from build123d import *

# Parameters (mm, degrees)
F0_R      = 40
F0_R_2    = 1.7
F1_DEPTH  = 14
F2_R      = 4.5
F2_R_2    = 1.7
F3_DEPTH  = 7
F4_R      = 4.5
F4_R_2    = 1.7
F5_DEPTH  = 4.6
F6_R      = 12.5
F7_DEPTH  = 8
F8_R      = 1
F10_R     = 32.1563127089
F11_DEPTH = 0.3


with BuildPart() as f1:
    # F0 (on Top) → F1 (new body)
    with BuildSketch(Plane.XY):
        Circle(F0_R)
        with Locations((-15.4640459878, -31.3984598617)):
            Circle(F0_R_2, mode=Mode.SUBTRACT)
        with Locations((-11.9054035877, -24.7893397535)):
            Circle(F0_R_2, mode=Mode.SUBTRACT)
        with Locations((-34.9238868738, -2.3069732602)):
            Circle(F0_R_2, mode=Mode.SUBTRACT)
        with Locations((-27.4208997634, -2.0842879275)):
            Circle(F0_R_2, mode=Mode.SUBTRACT)
        with Locations((19.4598408861, -29.0914866016)):
            Circle(F0_R_2, mode=Mode.SUBTRACT)
        with Locations((15.5154961757, -22.705051826)):
            Circle(F0_R_2, mode=Mode.SUBTRACT)
        with Locations((-15.5154961757, 22.705051826)):
            Circle(F0_R_2, mode=Mode.SUBTRACT)
        with Locations((-19.4598408861, 29.0914866016)):
            Circle(F0_R_2, mode=Mode.SUBTRACT)
        with Locations((27.4208997634, 2.0842879275)):
            Circle(F0_R_2, mode=Mode.SUBTRACT)
        with Locations((34.9238868738, 2.3069732602)):
            Circle(F0_R_2, mode=Mode.SUBTRACT)
        with Locations((11.9054035877, 24.7893397535)):
            Circle(F0_R_2, mode=Mode.SUBTRACT)
        with Locations((15.4640459878, 31.3984598617)):
            Circle(F0_R_2, mode=Mode.SUBTRACT)
    extrude(amount=F1_DEPTH)

    # F2 (on face) → F3 (cut)
    with BuildSketch(Plane.XY.offset(14)):
        with Locations((-15.5154961757, 22.705051826)):
            Circle(F2_R)
        with Locations((-15.5154961757, 22.705051826)):
            Circle(F2_R_2, mode=Mode.SUBTRACT)
        with Locations((-27.4208997634, -2.0842879275)):
            Circle(F2_R)
        with Locations((-27.4208997634, -2.0842879275)):
            Circle(F2_R_2, mode=Mode.SUBTRACT)
        with Locations((-11.9054035877, -24.7893397535)):
            Circle(F2_R)
        with Locations((-11.9054035877, -24.7893397535)):
            Circle(F2_R_2, mode=Mode.SUBTRACT)
        with Locations((15.5154961757, -22.705051826)):
            Circle(F2_R)
        with Locations((15.5154961757, -22.705051826)):
            Circle(F2_R_2, mode=Mode.SUBTRACT)
        with Locations((27.4208997634, 2.0842879275)):
            Circle(F2_R)
        with Locations((27.4208997634, 2.0842879275)):
            Circle(F2_R_2, mode=Mode.SUBTRACT)
        with Locations((11.9054035877, 24.7893397535)):
            Circle(F2_R)
        with Locations((11.9054035877, 24.7893397535)):
            Circle(F2_R_2, mode=Mode.SUBTRACT)
    extrude(amount=-F3_DEPTH, mode=Mode.SUBTRACT)

    # F4 (on face) → F5 (cut)
    with BuildSketch(Plane(origin=(0, 0, 0), x_dir=(1, 0, 0), z_dir=(0, 0, -1))):
        with Locations((27.4208997634, -2.0842879275)):
            Circle(F4_R)
        with Locations((27.4208997634, -2.0842879275)):
            Circle(F4_R_2, mode=Mode.SUBTRACT)
        with Locations((15.5154961757, 22.705051826)):
            Circle(F4_R)
        with Locations((15.5154961757, 22.705051826)):
            Circle(F4_R_2, mode=Mode.SUBTRACT)
        with Locations((-11.9054035877, 24.7893397535)):
            Circle(F4_R)
        with Locations((-11.9054035877, 24.7893397535)):
            Circle(F4_R_2, mode=Mode.SUBTRACT)
        with Locations((-27.4208997634, 2.0842879275)):
            Circle(F4_R)
        with Locations((-27.4208997634, 2.0842879275)):
            Circle(F4_R_2, mode=Mode.SUBTRACT)
        with Locations((-15.5154961757, -22.705051826)):
            Circle(F4_R)
        with Locations((-15.5154961757, -22.705051826)):
            Circle(F4_R_2, mode=Mode.SUBTRACT)
        with Locations((11.9054035877, -24.7893397535)):
            Circle(F4_R)
        with Locations((11.9054035877, -24.7893397535)):
            Circle(F4_R_2, mode=Mode.SUBTRACT)
        with Locations((27.4208997634, -2.0842879275)):
            Circle(F4_R_2)
    extrude(amount=-F5_DEPTH, mode=Mode.SUBTRACT)

    # F6 (on face) → F7 (cut)
    with BuildSketch(Plane.XY.offset(14)):
        Circle(F6_R)
    extrude(amount=-F7_DEPTH, mode=Mode.SUBTRACT)

    # F8
    f8_edges = [f1.edges().sort_by_distance(p)[0] for p in [
        (-12.5, 0, 6),
        (-12.5, 0, 14),
        (-40, 0, 14),
    ]]
    fillet(f8_edges, radius=F8_R)

    # F10 (on offset) → F11 (join)
    with BuildSketch(Plane(origin=(0, 0, 4.6), x_dir=(1, 0, 0), z_dir=(0, 0, -1))):
        Circle(F10_R)
    extrude(amount=-F11_DEPTH)


solid = f1.part
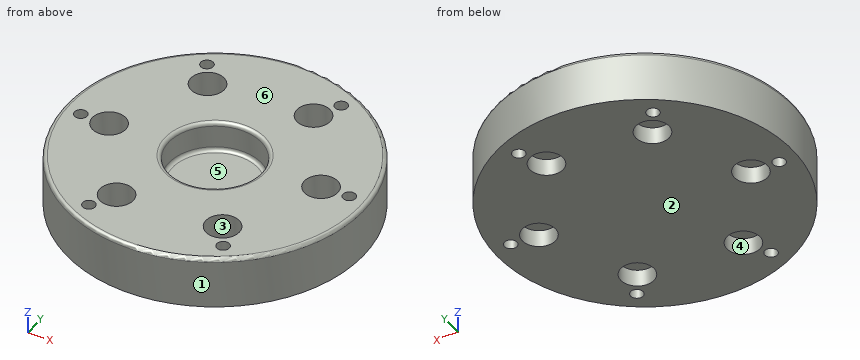
Verification items for the finished model (mm, model axes). Face numbers are marked on the shaded views. A direction names the side the tool comes from. Coordinates: 2 decimals unless noted, no trailing zeros. Order: outer loops, then holes, each group sorted by start corner. A loop starts at its lowest first (then second) coordinate and runs counter-clockwise, first axis right, second up.
1. Scan lines: line 1 (X direction, y = 21.5, z = 10.75); line 2 (Y direction, x = 13, z = 11); line 3 (Z direction, x = -2, y = 4). Record each from-to range of solid material in increasing order.
Results found:
line 1: x = -33.73 to -19.85, -11.18 to 8.83, 14.98 to 33.73
line 2: y = -37.83 to -26.44, -18.97 to 20.42, 29.15 to 37.83
line 3: z = 0 to 6
2. Release check for a two-part mould opening along X. For the marked faces 1, 2 and 3 record: +X half, -X half, draft (parallel to the pull), parting line (faces both ways), or undercut.
Results found:
face 1: parting line
face 2: draft
face 3: undercut
3. Set-up check for the marked faces 4, 5 and 6: record each of +Z, -Z, +X, -X, +Y, -Y from which the full face is reachable in a straight line by a thin tool's end or side.
Results found:
face 4: -Z
face 5: +Z
face 6: +Z, +X, -X, +Y, -Y
4. Sectioned sample at B-B, the plane x = 0. Record the cut outline in (y, z), and give its area (3 significant figures).
Results found:
outline: (-40, 0) - (40, 0) - (40, 13) arc R1 ccw to (39, 14) - (13.5, 14) arc R1 ccw to (12.5, 13) - (12.5, 7) arc R1 cw to (11.5, 6) - (-11.5, 6) arc R1 cw to (-12.5, 7) - (-12.5, 13) arc R1 ccw to (-13.5, 14) - (-39, 14) arc R1 ccw to (-40, 13) - close
area: 920 mm2
5. Sectioned sample at A-A, the plane z = 3. Give the number of separate pieces and of enclosed holes in the cut face, and give its area (3 significant figures).
Results found:
separate pieces: 1
enclosed holes: 12
area: 4,590 mm2
6. Go/stop test with flat-tipped pins: pin 1 Ø3 at (x, z) = (9, 1.5) entering from +Y; pin 2 Ø1 at (x, z) = (-9.5, 7) entering from +Y; pin 3 Ø1.5 at (x, z) = (16, 4) entering from +Y. Record where each tip stops, or that it passes through.
Results found:
pin 1: stops at y = 39.29
pin 2: stops at y = 38.97
pin 3: stops at y = 36.98
